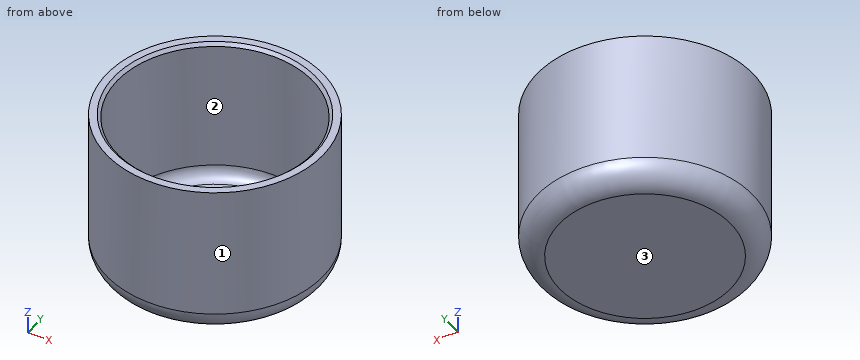
```python
from build123d import *

# Parameters (mm, degrees)
F0_W    = 8.75
F0_H    = 12.5
F2_R    = 1.8
F3_T    = -0.85
F4_SIZE = 0.25


with BuildPart() as f1:
    # F0 (on Front) → F1 (revolve)
    with BuildSketch(Plane.XZ):
        Rectangle(F0_W, F0_H)
    revolve(axis=Axis((-4.375, 0, 0), (0, 0, 1)))

    # F2
    f2_edges = [f1.edges().sort_by_distance(p)[0] for p in [
        (-13.125, 0, -6.25),
    ]]
    fillet(f2_edges, radius=F2_R)

    # F3
    f3_openings = [f1.faces().sort_by_distance(p)[0] for p in [
        (-4.375, 0, 6.25),
    ]]
    offset(amount=F3_T, openings=f3_openings)

    # F4
    f4_edges = [f1.edges().sort_by_distance(p)[0] for p in [
        (-12.275, 0, 6.25),
    ]]
    chamfer(f4_edges, length=F4_SIZE)


solid = f1.part
```
Check sheet for the modelled part. Datum: model origin and axes. Units: mm. Face numbers are marked on the shaded views. Coordinates: 2 decimals unless noted, no trailing zeros. Write each loop counter-clockwise with the first axis right and the second up, starting at its lowest first coordinate (ties: lowest second). Pieces come first, ordered by that corner, then holes. Notation, with made-up numbers: (-35, 13.5) -> (21, 13.5) arc R29 cw to (21, 52.5) -> close; hole circle Ø6 at (5, 85). An arc over 180 degrees is marked (long way). Use a Markdown table: item, result.
1. Sectioned sample at B-B (z = -0.5). Enter the section's corners in (x, y) (3 decimals), plus the area to 3 significant figures.
Reported:
| item | result |
|---|---|
| outline | circle Ø17.5 at (-4.375, 0); hole circle Ø15.8 at (-4.375, 0) |
| area | 44.5 mm2 |
2. Release check for a two-part mould opening along X. For the marked faces 1, 2 and 3 record: pulls with the +X half, pulls with the -X half, needs draft (parallel to the pull), parting line crosses it, or undercut.
Reported:
| item | result |
|---|---|
| face 1 | parting line crosses it |
| face 2 | undercut |
| face 3 | needs draft |
3. Scan lines: line 1 along X through (y, z) = (3.75, -3.5); line 2 along Z through (x, y) = (-4.25, -6); line 3 along Y through (x, z) = (-4.5, -4.75). Record each from-to range of solid material in increasing order.
Reported:
| item | result |
|---|---|
| line 1 | x = -12.28 to -11.33, 2.58 to 3.53 |
| line 2 | z = -6.25 to -5.4 |
| line 3 | y = -8.72 to -7.85, 7.85 to 8.72 |
4. Sectioned sample at A-A (y = 0). Enter the section's corners in (x, z) (3 decimals), plus the area to 3 significant figures.
Reported:
| item | result |
|---|---|
| outline | (-13.125, -4.45) arc R1.8 ccw to (-11.325, -6.25) -> (2.575, -6.25) arc R1.8 ccw to (4.375, -4.45) -> (4.375, 6.25) -> (3.775, 6.25) -> (3.525, 6) -> (3.525, -4.45) arc R0.95 cw to (2.575, -5.4) -> (-11.325, -5.4) arc R0.95 cw to (-12.275, -4.45) -> (-12.275, 6) -> (-12.525, 6.25) -> (-13.125, 6.25) -> close |
| area | 33.6 mm2 |
5. Go/stop test with flat-tipped pins: pin 1 Ø4 at (x, z) = (1, -3.5) entering from +Y; pin 2 Ø1 at (y, z) = (-7, 4) entering from -X; pin 3 Ø1.5 at (x, z) = (1.5, -2) entering from +Y. Record where each tip stops, or that it passes through.
Reported:
| item | result |
|---|---|
| pin 1 | stops at y = 8.07 |
| pin 2 | stops at x = -10.23 |
| pin 3 | stops at y = 7.09 |
